Model file for the job. Use its own axes, mm. Face numbers are marked on the shaded views. A direction names the side the tool comes from. Give positions to 0.01 mm unless a question says otherwise; leave off trailing zeros. Write each loop counter-clockwise with the first axis right and the second up, starting at its lowest first coordinate (ties: lowest second). Pieces come first, ordered by that corner, then holes. Notation, with made-up numbers: (-19.5, 32) - (20.5, 32) arc R18 cw to (20.5, 39) - close; hole circle Ø3 at (-31, 51). An arc over 180 degrees is marked (long way). Use CSV: the item, a comma, the result in double quotes.
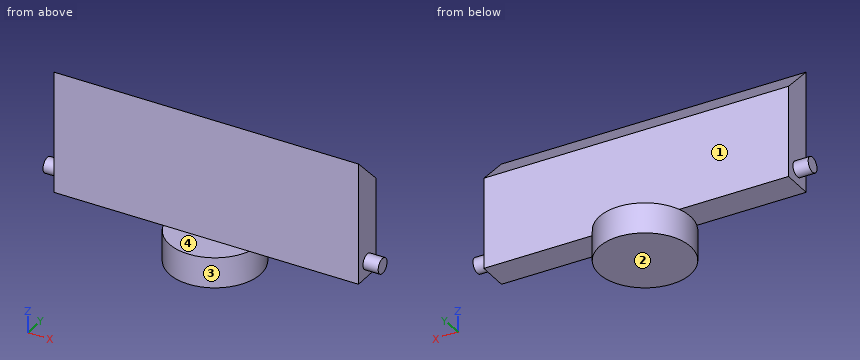
from build123d import *

# Parameters (mm, degrees)
BOSS_EXTRUDE1_DEPTH      = 4
BOSS_EXTRUDE1_DEPTH_BACK = 4
SKETCH2_W                = 20
SKETCH2_H                = 2
CUT_EXTRUDE1_DEPTH       = 20
SKETCH5_R                = 0.5
BOSS_EXTRUDE3_DEPTH      = 1
SKETCH8_R                = 3
BOSS_EXTRUDE5_DEPTH      = 2


with BuildPart() as part:
    # Sketch2 → Boss-Extrude1 (new, two sides: drawn at the far end of the back side and taken through both)
    with BuildSketch(Plane.XY.offset(-146.611129216).offset(-BOSS_EXTRUDE1_DEPTH_BACK)):
        with Locations((-43.541013266, -149.954890484)):
            Rectangle(SKETCH2_W, SKETCH2_H)
    extrude(amount=BOSS_EXTRUDE1_DEPTH + BOSS_EXTRUDE1_DEPTH_BACK)

    # Sketch4 → Cut-Extrude1 (cut)
    with BuildSketch(Plane.ZY.offset(53.541013266)):
        Polygon((-142.611129216, -148.954890484), (-142.611129216, -150.954890484), (-144.611129216, -148.954890484), align=None)
    extrude(amount=-CUT_EXTRUDE1_DEPTH, mode=Mode.SUBTRACT)

    # Sketch5 → Boss-Extrude3 (add)
    with BuildSketch(Plane.ZY.offset(53.541013266)):
        with Locations((-149.611129216, -149.954890484)):
            Circle(SKETCH5_R)
    boss_extrude3 = extrude(amount=BOSS_EXTRUDE3_DEPTH)

    # Mirror2: Boss-Extrude3 across plane
    add(boss_extrude3.mirror(Plane.ZY.offset(43.541013266)))

    # Sketch8 → Boss-Extrude5 (add)
    with BuildSketch(Plane(origin=(0, 0, -150.611129216), x_dir=(-1, 0, 0), z_dir=(0, 0, -1))):
        with Locations(Location((43.541013266, -149.954890484, 0), (0, 0, 199.471220634))):
            Circle(SKETCH8_R)
    extrude(amount=BOSS_EXTRUDE5_DEPTH)


solid = part.part
(1) Saw through at A-A, the plane z = -149.75. List the corners of the cut face in (x, y), then the cut area to 3 significant figures.
Checked values:
outline,"(-54.54, -150.44) - (-53.54, -150.44) - (-53.54, -150.95) - (-33.54, -150.95) - (-33.54, -150.44) - (-32.54, -150.44) - (-32.54, -149.47) - (-33.54, -149.47) - (-33.54, -148.95) - (-53.54, -148.95) - (-53.54, -149.47) - (-54.54, -149.47) - close"
area,"41.9 mm^2"
(2) Saw through at B-B, the plane x = -43.75. List the corners of the cut face in (y, z).
Checked values:
outline,"(-152.95, -152.61) - (-146.96, -152.61) - (-146.96, -150.61) - (-148.95, -150.61) - (-148.95, -144.61) - (-150.95, -142.61) - (-150.95, -150.61) - (-152.95, -150.61) - close"
(3) Flat gauge pins, fed straight in: P1, Ø1.6, axis at y = -149.5, z = -146.5, coming from the -X side; P2, Ø1.6, axis at x = -51, y = -150.5, coming from the -Z side; P3, Ø3, axis at x = -48.5, y = -148, coming from the +Z side. Where does each tip first touch, or does it go through?
Checked values:
P1,"stops at x = -53.54"
P2,"stops at z = -150.61"
P3,"stops at z = -144.07"
(4) Wall check: probe 1 along Y at (x, z) = (-38.75, -150); probe 2 along Z at (x, y) = (-45.25, -148); probe 3 along X at (y, z) = (-149.8, -144.25). Give the ranges that are in metal, low to high. Write a range as [from, to].
Checked values:
probe 1,"y = [-150.95, -148.95]"
probe 2,"z = [-152.61, -150.61]"
probe 3,"x = [-53.54, -33.54]"
(5) Saw through at D-D, the plane x = -47.75. List the corners of the cut face in (y, z), then the cut area to 3 significant figures.
Checked values:
outline,"(-150.95, -150.61) - (-148.95, -150.61) - (-148.95, -144.61) - (-150.95, -142.61) - close"
area,"14.0 mm^2"
(6) 3-axis set-ups, long thin cutter, end or side, ignore diameter. For the marked faces 1, 2, 3 and 4: which of +Z, -Z, +X, -X, +Y, -Y reach the whole face in a straight line?
Checked values:
face 1,"+Z, +X, -X, +Y"
face 2,"-Z, +X, -X, +Y, -Y"
face 3,"-Z"
face 4,"+Z, +X, -X, -Y"
(7) Saw through at C-C, the plane y = -147.45. List the corners of the cut face in (x, z).
Checked values:
outline,"(-45.19, -152.61) - (-41.89, -152.61) - (-41.89, -150.61) - (-45.19, -150.61) - close"
